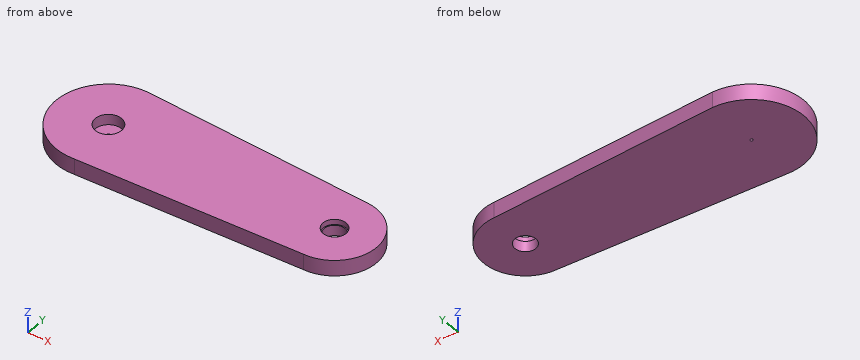
```python
from build123d import *

# Parameters (mm, degrees)
CROQUIS1_R              = 1.25
CROQUIS1_R_2            = 10
SALIENTE_EXTRUIR1_DEPTH = 15
CROQUIS2_R              = 12.5
CORTAR_EXTRUIR1_DEPTH   = 10
CROQUIS3_R              = 11
CORTAR_EXTRUIR2_DEPTH   = 5


with BuildPart() as part:
    # Croquis1 → Saliente-Extruir1 (new body)
    with BuildSketch(Plane.XY):
        with BuildLine():
            Line((0, 50), (215, 40))
            ThreePointArc((215, 40), (255, 0), (215, -40))
            Line((215, -40), (4.641122504, -49.784133837))
            ThreePointArc((4.641122504, -49.784133837), (-49.946004304, -2.323069968), (0, 50))
        make_face()
        Circle(CROQUIS1_R, mode=Mode.SUBTRACT)
        with Locations((215, 0)):
            Circle(CROQUIS1_R_2, mode=Mode.SUBTRACT)
    extrude(amount=SALIENTE_EXTRUIR1_DEPTH)

    # Croquis2 → Cortar-Extruir1 (cut)
    with BuildSketch(Plane.XY.offset(15)):
        Circle(CROQUIS2_R)
    extrude(amount=-CORTAR_EXTRUIR1_DEPTH, mode=Mode.SUBTRACT)

    # Croquis3 → Cortar-Extruir2 (cut)
    with BuildSketch(Plane.XY.offset(15)):
        with Locations((215, 0)):
            Circle(CROQUIS3_R)
    extrude(amount=-CORTAR_EXTRUIR2_DEPTH, mode=Mode.SUBTRACT)


solid = part.part
```
Input: part model. Units: mm. Frame: model coordinates. Coordinates: 2 decimals unless noted, no trailing zeros. Loops run counter-clockwise (first coordinate to the right, second up) from the corner with the lowest first, then second, coordinate; pieces in that order, holes last. Notation, with made-up numbers: (78, -9.75) -> (114, -9.75) arc R17 ccw to (114, -4.75) -> close; hole circle Ø2 at (-12.75, -6.75). An arc over 180 degrees is marked (long way). Use a Markdown table: item, result.
1) Cut plane B-B (y = -33). Return the cut outline in (x, z).
Results found:
| item | result |
|---|---|
| outline | (-37.56, 0) -> (237.61, 0) -> (237.61, 15) -> (-37.56, 15) -> close |
2) Contact query for flat-ended pins moving along their axis: pin 1 (2 mm diameter, centred on x = 21, z = 4, fed in from +Y); pin 2 (3 mm diameter, centred on x = -17.5, z = 10, fed in from +Y); pin 3 (12.5 mm diameter, centred on x = 3, y = -2.5, fed in from +Z). Output: stop coordinate, or through.
Results found:
| item | result |
|---|---|
| pin 1 | stops at y = 49.07 |
| pin 2 | stops at y = 47.37 |
| pin 3 | stops at z = 5 |
3) Cut plane A-A (x = 43.5). Return the cut outline in (y, z), then the cut area to 3 significant figures.
Results found:
| item | result |
|---|---|
| outline | (-47.98, 0) -> (47.98, 0) -> (47.98, 15) -> (-47.98, 15) -> close |
| area | 1,440 mm2 |
4) Material intervals for line 1 along Y through (x, z) = (215, 2.75); line 2 along Y through (x, z) = (0, 9.75); line 3 along X through (y, z) = (2, 9), sorted ascending. Write a range as from..to.
Results found:
| item | result |
|---|---|
| line 1 | y = -40..-10, 10..40 |
| line 2 | y = -50..-12.5, 12.5..50 |
| line 3 | x = -49.96..-12.34, 12.34..205.2, 224.8..254.95 |
